```python
from build123d import *
from build123d.topology import SkipClean

# Parameters (mm, degrees)
SKETCH1_R           = 38.1
SKETCH1_R_2         = 19.05
BOSS_EXTRUDE1_DEPTH = 63.5
BOSS_EXTRUDE2_START = -12.7
SKETCH1_3_R         = 139.7
SKETCH1_3_R_2       = 101.6
SKETCH1_3_R_3       = 38.1
SKETCH1_3_R_4       = 19.05
BOSS_EXTRUDE2_DEPTH = 12.7
BOSS_EXTRUDE3_START = 165.1
BOSS_EXTRUDE3_DEPTH = 165.1
CIRPATTERN2_COUNT   = 6
BOSS_EXTRUDE4_START = 6.35
SKETCH3_R           = 139.7
SKETCH3_R_2         = 101.6
BOSS_EXTRUDE4_DEPTH = 6.35


with BuildPart() as part:
    # Sketch1 → Boss-Extrude1 (new body)
    with BuildSketch(Plane.XY):
        Circle(SKETCH1_R)
        Circle(SKETCH1_R_2, mode=Mode.SUBTRACT)
    extrude(amount=BOSS_EXTRUDE1_DEPTH)

    # Sketch1_3 → Boss-Extrude2 (add)
    # profile 1 of 3: a face of its own
    with BuildSketch(Plane.XY.offset(BOSS_EXTRUDE2_START)):
        Circle(SKETCH1_3_R)
        Circle(SKETCH1_3_R_2, mode=Mode.SUBTRACT)
    # profile 2 of 3: a face of its own
    with BuildSketch(Plane.XY.offset(BOSS_EXTRUDE2_START)):
        Circle(SKETCH1_3_R_2)
        Circle(SKETCH1_3_R_3, mode=Mode.SUBTRACT)
    # profile 3 of 3: a face of its own
    with BuildSketch(Plane.XY.offset(BOSS_EXTRUDE2_START)):
        Circle(SKETCH1_3_R_3)
        Circle(SKETCH1_3_R_4, mode=Mode.SUBTRACT)
    extrude(amount=BOSS_EXTRUDE2_DEPTH)

    # Sketch2 → Boss-Extrude3 (add)
    with SkipClean():  # the faces are left unmerged after this step: merging them gives an invalid solid
        with BuildSketch(Plane(origin=(0, 0, -12.7), x_dir=(-1, 0, 0), z_dir=(0, 0, -1)).offset(BOSS_EXTRUDE3_START)):
            with BuildLine():
                Line((-107.016408704, 89.797429073), (-104.097779375, 87.34840828))
                ThreePointArc((-104.097779375, 87.34840828), (-89.757405887, 102.027938274), (-73.370038531, 114.380634489))
                Line((-73.370038531, 114.380634489), (-75.277064912, 117.683701073))
                ThreePointArc((-75.277064912, 117.683701073), (-92.207042422, 104.947374087), (-107.016408704, 89.797429073))
            make_face()
            with BuildLine():
                ThreePointArc((-73.370038531, 114.380634489), (-70.676823655, 116.064114601), (-67.945, 117.68419212))
                Line((-67.945, 117.68419212), (-69.85, 120.983748909))
                ThreePointArc((-69.85, 120.983748909), (-72.582289999, 119.364572544), (-75.277064912, 117.683701073))
                Line((-75.277064912, 117.683701073), (-73.370038531, 114.380634489))
            make_face()
            with BuildLine():
                Line((-43.599261314, 62.816135768), (-38.1, 65.991135768))
                Line((-38.1, 65.991135768), (-67.945, 117.68419212))
                ThreePointArc((-67.945, 117.68419212), (-70.676823655, 116.064114601), (-73.370038531, 114.380634489))
                Line((-73.370038531, 114.380634489), (-43.599261314, 62.816135768))
            make_face()
        boss_extrude3 = extrude(amount=-BOSS_EXTRUDE3_DEPTH)

    # CirPattern2: Boss-Extrude3 ×6 about axis
    with SkipClean():  # the faces are left unmerged after this step: merging them gives an invalid solid
        cirpattern2_axis = Axis((0, 0, 0), (0, 0, 1))
        for i in range(1, CIRPATTERN2_COUNT):
            add(boss_extrude3.rotate(cirpattern2_axis, i * 360 / CIRPATTERN2_COUNT))

    # Sketch3 → Boss-Extrude4 (add)
    with SkipClean():  # the faces are left unmerged after this step: merging them gives an invalid solid
        with BuildSketch(Plane(origin=(0, 0, -177.8), x_dir=(-1, 0, 0), z_dir=(0, 0, -1)).offset(BOSS_EXTRUDE4_START)):
            with Locations(Location((0, 0, 0), (0, 0, 180))):
                Circle(SKETCH3_R)
            Circle(SKETCH3_R_2, mode=Mode.SUBTRACT)
        extrude(amount=-BOSS_EXTRUDE4_DEPTH)


solid = part.part
```
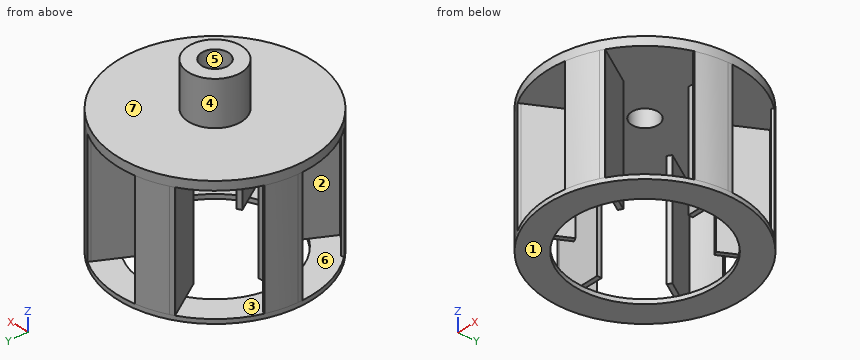
Here's how the part is built. I have some questions about the finished solid (model axes, mm). Face numbers are marked on the shaded views. A direction names the side the tool comes from. Give positions to 0.01 mm unless a question says otherwise; leave off trailing zeros. Order: outer loops, then holes, each group sorted by start corner. A loop starts at its lowest first (then second) coordinate and runs counter-clockwise, first axis right, second up. Notation, with made-up numbers: (74.25, -4) -> (122.25, -4) arc R14 cw to (122.25, 13) -> close; hole circle Ø9 at (23, 22). An arc over 180 degrees is marked (long way). Use CSV: the item, a comma, the result in double quotes. Start each with the question number.
Item 1: I'm going to push flat-ended pins straight in: P1, Ø25, axis at x = 118, y = 43.5, coming from the +Z side; P2, Ø7, axis at y = 2.5, z = -110, coming from the +X side; P3, Ø12, axis at y = -81.5, z = 11, coming from the +X side; P4, Ø20, axis at x = -45, y = 72.5, coming from the -Z side. Where does each tip first touch, or does it pass through?
Item 2: Suppose I cut it at B-B (y = -29). List the corners of the cut face in (x, z) for me, and give its area (3 significant figures).
Item 3: Suppose I cut it at C-C (x = 95). List the corners of the cut face in (y, z) for me.
Item 4: If I drill on probe 1 along Z at (x, y) = (116.5, 34); probe 2 along Y at (x, z) = (0, 36.5); probe 3 along Y at (x, z) = (-46, -92), over which ranges is the centre line in solid material (lowest first)? Write a range as [from, to].
Item 5: Suppose I cut it at D-D (z = -36). Give the number of separate pieces and of enclosed holes in the cut face, and give its area (3 significant figures).
Item 6: On a 3-axis mill with a long thin cutter (end or side, diameter ignored), from which of +Z, -Z, +X, -X, +Y, -Y can I reach the whole of each face in a straight line? I mean the marked faces 5, 6 and 7. Say none if no direction works.
Item 7: Suppose I cut it at A-A (x = 0). List the corners of the cut face in (y, z) for me.
Item 8: Thinking about a two-plate mould opening in Z: for the marked faces 1, 2, 3 and 4, which applies, pulls with the +Z half, pulls with the -Z half, needs draft (parallel to the pull), parting line crosses it, or undercut?
Answer block:
1,P1,"stops at z = 0"
1,P2,"stops at x = 139.7"
1,P3,"passes through"
1,P4,"stops at z = -177.8"
2,outline,"(-136.66, -184.15) -> (-97.37, -184.15) -> (-97.37, -177.8) -> (-136.66, -177.8) -> close; (-136.66, -12.7) -> (132.76, -12.7) -> (132.76, -177.8) -> (97.37, -177.8) -> (97.37, -184.15) -> (136.66, -184.15) -> (136.66, 0) -> (24.71, 0) -> (24.71, 63.5) -> (-24.71, 63.5) -> (-24.71, 0) -> (-136.66, 0) -> close"
2,area,"7,750 mm^2"
3,outline,"(-102.43, -184.15) -> (-36.02, -184.15) -> (-36.02, -177.8) -> (-102.43, -177.8) -> close; (-102.43, -12.7) -> (-6.35, -12.7) -> (-6.35, -177.8) -> (0, -177.8) -> (0, -12.7) -> (97.17, -12.7) -> (97.17, -177.8) -> (36.02, -177.8) -> (36.02, -184.15) -> (102.43, -184.15) -> (102.43, 0) -> (-102.43, 0) -> close"
4,probe 1,"z = [-184.15, -177.8], [-12.7, 0]"
4,probe 2,"y = [-38.1, -19.05], [19.05, 38.1]"
4,probe 3,"y = [-79.67, -66.97], [79.67, 92.37], [127.87, 131.91]"
5,separate pieces,"6"
5,enclosed holes,"0"
5,area,"3,370 mm^2"
6,face 5,"+Z, -Z"
6,face 6,"none"
6,face 7,"+Z"
7,outline,"(-139.7, -184.15) -> (-101.6, -184.15) -> (-101.6, -177.8) -> (-139.7, -177.8) -> close; (-139.7, -12.7) -> (-19.05, -12.7) -> (-19.05, 63.5) -> (-38.1, 63.5) -> (-38.1, 0) -> (-139.7, 0) -> close; (19.05, -12.7) -> (139.7, -12.7) -> (139.7, 0) -> (38.1, 0) -> (38.1, 63.5) -> (19.05, 63.5) -> close; (101.6, -184.15) -> (139.7, -184.15) -> (139.7, -177.8) -> (101.6, -177.8) -> close"
8,face 1,"pulls with the -Z half"
8,face 2,"undercut"
8,face 3,"undercut"
8,face 4,"needs draft"
